from build123d import *

# Parameters (mm, degrees)
BOSS_EXTRUDE1_DEPTH = 11.43
FILLET1_R           = 5.715
SKETCH3_R           = 2.2225
SKETCH3_R_2         = 1.905
CUT_EXTRUDE1_DEPTH  = 12.7
FILLET2_R           = 2.54


with BuildPart() as part:
    # Sketch1 → Boss-Extrude1 (new body)
    with BuildSketch(Plane.XY):
        Polygon((0, 0), (0, 20.102102448), (9.525, 29.627102448), (9.525, 51.852102448), (12.065, 51.852102448), (12.065, 28.575), (2.54, 19.05), (2.54, 0), align=None)
    extrude(amount=BOSS_EXTRUDE1_DEPTH)

    # Fillet1
    fillet1_edges = [part.edges().sort_by_distance(p)[0] for p in [
        (10.795, 51.852102448, 0),
        (10.795, 51.852102448, 11.43),
    ]]
    fillet(fillet1_edges, radius=FILLET1_R - 0.0001)  # a hair under: the kernel refuses the full size

    # Sketch3 → Cut-Extrude1 (cut)
    with BuildSketch(Plane(origin=(12.065, 0, 0), x_dir=(0, 0, -1), z_dir=(1, 0, 0))):
        with Locations(Location((-5.715, 46.137102448, 0), (0, 0, 90))):
            Circle(SKETCH3_R)
        with Locations((-5.715, 8.89)):
            Circle(SKETCH3_R_2)
    extrude(amount=-CUT_EXTRUDE1_DEPTH, mode=Mode.SUBTRACT)

    # Fillet2
    fillet2_edges = [part.edges().sort_by_distance(p)[0] for p in [
        (0, 20.102102448, 5.715),
        (9.525, 29.627102448, 5.715),
        (12.065, 28.575, 5.715),
        (2.54, 19.05, 5.715),
    ]]
    fillet(fillet2_edges, radius=FILLET2_R)


solid = part.part
Part model, mm, in its own coordinate system. A direction names the side the tool comes from. Give positions to 0.01 mm unless a question says otherwise; leave off trailing zeros. Loops run counter-clockwise (first coordinate to the right, second up) from the corner with the lowest first, then second, coordinate; pieces in that order, holes last.
(1) Band-saw the part on C-C (z = 10.25). Write the cut outline in (x, y) (3 decimals), and give its area (3 significant figures).
Return value:
outline: (0, 0) - (2.54, 0) - (2.54, 17.998) arc R2.54 cw to (3.284, 19.794) - (11.321, 27.831) arc R2.54 ccw to (12.065, 29.627) - (12.065, 49.615) - (9.525, 49.615) - (9.525, 30.679) arc R2.54 cw to (8.781, 28.883) - (0.744, 20.846) arc R2.54 ccw to (0, 19.05) - close
area: 136 mm2
(2) Band-saw the part on A-A (y = 8.89). Write the cut outline in (x, z), and give its area (3 significant figures).
Return value:
outline: (0, 0) - (2.54, 0) - (2.54, 3.81) - (0, 3.81) - close; (0, 7.62) - (2.54, 7.62) - (2.54, 11.43) - (0, 11.43) - close
area: 19.4 mm2
(3) Drill centre lines: line 1 along Y through (x, z) = (11.25, 7.5); line 2 along X through (y, z) = (5.5, 10.75); line 3 along X through (y, z) = (40, 8) (3 decimals). Where is each one in solid material? Low to high.
Return value:
line 1: y = 27.76 to 44.81, 47.46 to 51.57
line 2: x = 0 to 2.54
line 3: x = 9.525 to 12.065
(4) Band-saw the part on D-D (y = 37). Write the cut outline in (x, z) (3 decimals), and give its area (3 significant figures).
Return value:
outline: (9.525, 0) - (12.065, 0) - (12.065, 11.43) - (9.525, 11.43) - close
area: 29.0 mm2
(5) 3-axis set-ups, long thin cutter, end or side, ignore diameter. For faces 1 (the flat face through (2.54, 11, 6)), 2 (the cylindrical face through (10.813, 50.222, 9.711)), 3 (the flat face through (9.525, 41, 6)): which of +Z, -Z, +X, -X, +Y, -Y reach the whole face in a straight line?
Return value:
face 1: +Z, -Z, +X, -Y
face 2: +Z, +X, -X, +Y
face 3: +Z, -Z, -X, +Y
(6) Pin check, flat tips, straight feed: pin 1 (5 mm diameter, centred on y = 8.89, z = 5.715, fed in from -X); pin 2 (6 mm diameter, centred on x = 7, y = 17, fed in from +Z). Stop position of each tip, or through.
Return value:
pin 1: stops at x = 0
pin 2: passes through
